from build123d import *

# Parameters (mm, degrees)
ESTRUSIONE_SOTTILE1_DEPTH                    = 10
SCHIZZO4_W                                   = 20
SCHIZZO4_H                                   = 50
ESTRUSIONE_ESTRUSIONE1_DEPTH                 = 2
SCHIZZO1_W                                   = 20
SCHIZZO1_H                                   = 165
ESTRUSIONE_ESTRUSIONE2_DEPTH                 = 2
RACCORDO2_R                                  = 10
RACCORDO8_R                                  = 2
LOFT3_START                                  = -1.559581264
LOFT3_OUTLINE_W                              = 20
LOFT3_OUTLINE_H                              = 2.50416156
LOFT3_DEPTH                                  = 1.559581264
RACCORDO13_R                                 = 2
RACCORDO14_R                                 = 2
FORO_FILETTATO_G1_16_2_AT_2_COUNT            = 2
FORO_FILETTATO_G1_16_2_AT_2_PITCH            = 110.419904734
FORO_LAMATO_PER_BULLONE_M3_A_TESTA_E_2_COUNT = 2
FORO_LAMATO_PER_BULLONE_M3_A_TESTA_E_2_PITCH = 10.95


with BuildPart() as part:
    # Schizzo5 → Estrusione-Sottile1 (new, symmetric)
    with BuildSketch(Plane(origin=(0, 0, 0), x_dir=(0, 0, -1), z_dir=(1, 0, 0))):
        Polygon((-20, -4.427601882), (0, 0), (0.43229372, -1.952721726), (-19.56770628, -6.380323609), align=None)
    extrude(amount=ESTRUSIONE_SOTTILE1_DEPTH, both=True)

    # Schizzo4 → Estrusione-Estrusione1 (add)
    with BuildSketch(Plane.XY.offset(20)):
        with Locations((0, -29.427601882)):
            Rectangle(SCHIZZO4_W, SCHIZZO4_H)
    extrude(amount=-ESTRUSIONE_ESTRUSIONE1_DEPTH)

    # Raccordo2
    raccordo2_edges = [part.edges().sort_by_distance(p)[0] for p in [
        (0, -6.033264645, 18),
    ]]
    fillet(raccordo2_edges, radius=RACCORDO2_R)

    # Raccordo8
    raccordo8_edges = [part.edges().sort_by_distance(p)[0] for p in [
        (0, -4.427601882, 20),
    ]]
    fillet(raccordo8_edges, radius=RACCORDO8_R)



with BuildPart() as body_2:
    # Schizzo1 → Estrusione-Estrusione2 (new body)
    with BuildSketch(Plane.XY):
        with Locations((0, 82.5)):
            Rectangle(SCHIZZO1_W, SCHIZZO1_H)
    extrude(amount=-ESTRUSIONE_ESTRUSIONE2_DEPTH)


with BuildPart() as part_1:
    add(part.part)

    add(body_2.part)  # Loft3 merges body 2
    # Loft3: read off the stored shape, not the designer's step
    # Loft3 outline → Loft3 (add)
    with BuildSketch(Plane(origin=(0, 0, 0), x_dir=(1, 0, 0), z_dir=(0, 0.626040390160855, 0.779790632084821)).offset(LOFT3_START)):
        Rectangle(LOFT3_OUTLINE_W, LOFT3_OUTLINE_H)
    extrude(amount=LOFT3_DEPTH)

    # Raccordo13
    raccordo13_edges = [part_1.edges().sort_by_distance(p)[0] for p in [
        (0, -1.952721726, -0.43229372),
    ]]
    fillet(raccordo13_edges, radius=RACCORDO13_R)

    # Raccordo14
    raccordo14_edges = [part_1.edges().sort_by_distance(p)[0] for p in [
        (0, 0, 0),
    ]]
    fillet(raccordo14_edges, radius=RACCORDO14_R)

    # Schizzo11 → Foro filettato G1/16-2 (revolve, cut)
    with BuildSketch(Plane(origin=(0, 146.829705844, 0), x_dir=(0, -1, 0), z_dir=(1, 0, 0))):
        Polygon((0, 0), (0, 2.005), (3.3, 2.005), (3.3, 0.5865), (3.8865, 0), align=None)
    foro_filettato_g1_16_2 = revolve(axis=Axis((0, 146.829705844, 6.35), (0, 0, -1)), mode=Mode.SUBTRACT)

    # Foro filettato G1/16-2 at 2: Foro filettato G1/16-2 ×2
    with Locations(*[(0, -i * FORO_FILETTATO_G1_16_2_AT_2_PITCH, 0) for i in range(1, FORO_FILETTATO_G1_16_2_AT_2_COUNT)]):
        add(foro_filettato_g1_16_2, mode=Mode.SUBTRACT)

    # Schizzo27 → Foro lamato per Bullone M3 a testa esagonale-4 (revolve, cut)
    with BuildSketch(Plane(origin=(0, -26.530198891, 20), x_dir=(0, -1, 0), z_dir=(1, 0, 0))):
        Polygon((0, 0), (0, 22.005), (1.7, 22.005), (1.7, 0.5), (4.5, 0.5), (4.5, 0.025), (4.525, 0), align=None)
    foro_lamato_per_bullone_m3_a_testa_esago = revolve(axis=Axis((0, -26.530198891, 26.35), (0, 0, -1)), mode=Mode.SUBTRACT)

    # Foro lamato per Bullone M3 a testa e 2: Foro lamato per Bullone M3 a testa esagonale-4 ×2
    with Locations(*[(0, -i * FORO_LAMATO_PER_BULLONE_M3_A_TESTA_E_2_PITCH, 0) for i in range(1, FORO_LAMATO_PER_BULLONE_M3_A_TESTA_E_2_COUNT)]):
        add(foro_lamato_per_bullone_m3_a_testa_esago, mode=Mode.SUBTRACT)


solid = part_1.part
Work out the finished part from the listing and answer in its coordinate system (mm). A direction names the side the tool comes from. Round coordinates to 2 decimals unless told otherwise and drop trailing zeros. Loops run counter-clockwise (first coordinate to the right, second up) from the corner with the lowest first, then second, coordinate; pieces in that order, holes last. Notation, with made-up numbers: (5.5, 18) - (26.5, 18) arc R26 cw to (26.5, 42) - close; hole circle Ø6 at (-12, -11.5). An arc over 180 degrees is marked (long way). One line per item, written item: value.
Q1. The mould has two halves that part along X. Classify faces 6 (the cylindrical face through (1.26, 33.36, -1.28)), 7 (the flat face through (-10, 39, -1)), 8 (the flat face through (0.14, -3.186, 5.139)): +X half, -X half, draft (parallel to the pull), parting line (faces both ways), or undercut.
Check values:
face 6: undercut
face 7: -X half
face 8: draft
Q2. Straight lines are drawn through the part: probe 1 along Y at (x, z) = (0, -1.3); probe 2 along Y at (x, z) = (0, -1.5); probe 3 along Z at (x, y) = (-6.25, 4). For each, find the intervals that lie inside material, in ascending order.
Check values:
probe 1: -0.87 to 33.11, 39.71 to 143.53, 150.13 to 165
probe 2: -0.62 to 33.11, 39.71 to 143.53, 150.13 to 165
probe 3: -2 to 0
Q3. Find section B-B on z = 12.25. Give the vertices of the cut face in (x, y), and give its area (3 significant figures).
Check values:
outline: (-10, -5.01) - (10, -5.01) - (10, -2.71) - (-10, -2.71) - close
area: 46.0 mm2
Q4. Find section A-A on y = 51. Give the vertices of the cut face in (x, z).
Check values:
outline: (-10, -2) - (10, -2) - (10, 0) - (-10, 0) - close
Q5. For faces 1 (the flat face through (0, 84, -2)), 2 (the flat face through (0, -34, 18)), 3 (the flat face through (4, -30, 20)), 4 (the flat face through (0, 84, 0)), 5 (the flat face through (-0.1, -24.6, 19.5)), determine the directions among +Z, -Z, +X, -X, +Y, -Y from which every point of the face is accessible in a straight line to the end or side of a thin tool.
Check values:
face 1: -Z, +X, -X, +Y, -Y
face 2: -Z, +X, -X, -Y
face 3: +Z, +X, -X, +Y, -Y
face 4: +Z, +X, -X, +Y
face 5: +Z
Q6. Each of these flat-tipped pins is pushed along its axis until it touches: pin 1 Ø2 at (x, z) = (-4.5, 1.5) entering from +Y; pin 2 Ø6 at (x, y) = (-1, 117) entering from +Z; pin 3 Ø5.5 at (x, y) = (0, -26.53) entering from -Z. Where does it stop, or does it pass through?
Check values:
pin 1: y = 0.28
pin 2: z = 0
pin 3: z = 18
